```python
from build123d import *

# Parameters (mm, degrees)
BASE_FLANGE1_DEPTH = 10
SKETCH6_R          = 1.984375
CUT_EXTRUDE1_DEPTH = 34.421549934


# Sheet-metal steps are written as plain solids
with BuildPart() as part:
    # Sketch1 → Base-Flange1 (new, symmetric)
    with BuildSketch(Plane(origin=(0, 0, 0), x_dir=(0, 0, -1), z_dir=(1, 0, 0))):
        with BuildLine():
            Line((-21, 0), (-13.4732, 0))
            ThreePointArc((-13.4732, 0), (-12.43149029, 0.43149029), (-12, 1.4732))
            Line((-12, 1.4732), (-12, 12))
            ThreePointArc((-12, 12), (0, 24), (12, 12))
            Line((12, 12), (12, 1.4732))
            ThreePointArc((12, 1.4732), (12.43149029, 0.43149029), (13.4732, 0))
            Line((13.4732, 0), (21, 0))
            Line((21, 0), (21, 0.7366))
            Line((21, 0.7366), (13.4732, 0.7366))
            ThreePointArc((13.4732, 0.7366), (12.952345145, 0.952345145), (12.7366, 1.4732))
            Line((12.7366, 1.4732), (12.7366, 12))
            ThreePointArc((12.7366, 12), (0, 24.7366), (-12.7366, 12))
            Line((-12.7366, 12), (-12.7366, 1.4732))
            ThreePointArc((-12.7366, 1.4732), (-12.952345145, 0.952345145), (-13.4732, 0.7366))
            Line((-13.4732, 0.7366), (-21, 0.7366))
            Line((-21, 0.7366), (-21, 0))
        make_face()
    extrude(amount=BASE_FLANGE1_DEPTH, both=True)

    # Sketch6 → Cut-Extrude1 (cut, through all)
    with BuildSketch(Plane(origin=(0, 0.7366, 0), x_dir=(1, 0, 0), z_dir=(0, 1, 0))):
        with Locations(Location((0, -17, 0), (0, 0, 270))):
            Circle(SKETCH6_R)
    cut_extrude1 = extrude(amount=-CUT_EXTRUDE1_DEPTH, mode=Mode.SUBTRACT)

    # Mirror1: Cut-Extrude1 across plane
    add(cut_extrude1.mirror(Plane.XY), mode=Mode.SUBTRACT)


solid = part.part
```
Can you work these out from the model? Positions are in its coordinate system, mm. A direction names the side the tool comes from. Give positions to 0.01 mm unless a question says otherwise; leave off trailing zeros. Loops run counter-clockwise (first coordinate to the right, second up) from the corner with the lowest first, then second, coordinate; pieces in that order, holes last. Notation, with made-up numbers: M 49.25,-14 L 77.25,-14 A23 cw 77.25,-2 Z; hole C 43,12.5 d11. An arc over 180 degrees is marked long. Use one line per item in the form item = value. Start each with the question number.
(1) I want a section at C-C, the plane z = 17. Write out the boundary of the cut face in (x, y), and give its area (3 significant figures).
(2) I want a section at B-B, the plane y = 9.25. Write out the boundary of the cut face in (x, z).
(3) Thinking about a two-plate mould opening in Z: for faces 4 (the cylindrical face through (0.6, 0.37, -18.89)), 5 (the flat face through (0, 7, 12.737)), 6 (the cylindrical face through (0.14, 0.42, 12.443)), 7 (the flat face through (2.4, 0.737, 17.2)), which applies, released by +Z, released by -Z, zero draft, split by the parting line, or undercut?
(4) I'm going to push flat-ended pins straight in: P1, Ø8.5, axis at x = 0.5, y = 8.5, coming from the +Z side; P2, Ø12, axis at x = 0, z = -10.5, coming from the +Y side; P3, Ø8.5, axis at x = 0, y = 7, coming from the -Z side; P4, Ø2.5, axis at x = 0, z = 17, coming from the +Y side. Where does each tip first touch, or does it pass through?
(5) Please list where these lines run through material, in increasing order: line 1 (X direction, y = 0.35, z = 17); line 2 (Z direction, x = -1, y = 9); line 3 (Y direction, x = -4.5, z = 0).
(6) I want a section at A-A, the plane x = 0. Write out the boundary of the cut face in (y, z), and give its area (3 significant figures).
(7) I want a section at D-D, the plane x = -6.5. Write out the boundary of the cut face in (y, z).
(8) On a 3-axis mill with a long thin cutter (end or side, diameter ignored), from which of +Z, -Z, +X, -X, +Y, -Y can I reach the whole of each face in a straight line? I mean faces 1 (the flat face through (0, 7, 12)), 2 (the flat face through (2.4, 0.737, -17.3)), 3 (the flat face through (2.4, 0, 17.3)). Say none if no direction works.
Worked out:
q1.outline = M -10,0 L -1.98,0 L -1.98,0.74 L -10,0.74 Z; M 1.98,0 L 10,0 L 10,0.74 L 1.98,0.74 Z
q1.area = 11.8 mm²
q2.outline = M -10,-12.74 L 10,-12.74 L 10,-12 L -10,-12 Z; M -10,12 L 10,12 L 10,12.74 L -10,12.74 Z
q3.face_4 = undercut
q3.face_5 = released by +Z
q3.face_6 = undercut
q3.face_7 = zero draft
q4.P1 = 12.74
q4.P2 = 23.92
q4.P3 = -12.74
q4.P4 = through
q5.line_1 = -10 to -1.98, 1.98 to 10
q5.line_2 = -12.74 to -12, 12 to 12.74
q5.line_3 = 24 to 24.74
q6.outline = M 0,-21 L 0.74,-21 L 0.74,-18.98 L 0,-18.98 Z; M 0,-15.02 L 0.74,-15.02 L 0.74,-13.47 A0.74 cw 1.47,-12.74 L 12,-12.74 A12.74 ccw 12,12.74 L 1.47,12.74 A0.74 cw 0.74,13.47 L 0.74,15.02 L 0,15.02 L 0,13.47 A1.47 ccw 1.47,12 L 12,12 A12 cw 12,-12 L 1.47,-12 A1.47 ccw 0,-13.47 Z; M 0,18.98 L 0.74,18.98 L 0.74,21 L 0,21 Z
q6.area = 51.9 mm²
q7.outline = M 0,-21 L 0.74,-21 L 0.74,-13.47 A0.74 cw 1.47,-12.74 L 12,-12.74 A12.74 ccw 12,12.74 L 1.47,12.74 A0.74 cw 0.74,13.47 L 0.74,21 L 0,21 L 0,13.47 A1.47 ccw 1.47,12 L 12,12 A12 cw 12,-12 L 1.47,-12 A1.47 ccw 0,-13.47 Z
q8.face_1 = +X, -X, -Y
q8.face_2 = -Z, +X, -X, +Y
q8.face_3 = +Z, -Z, +X, -X, -Y
